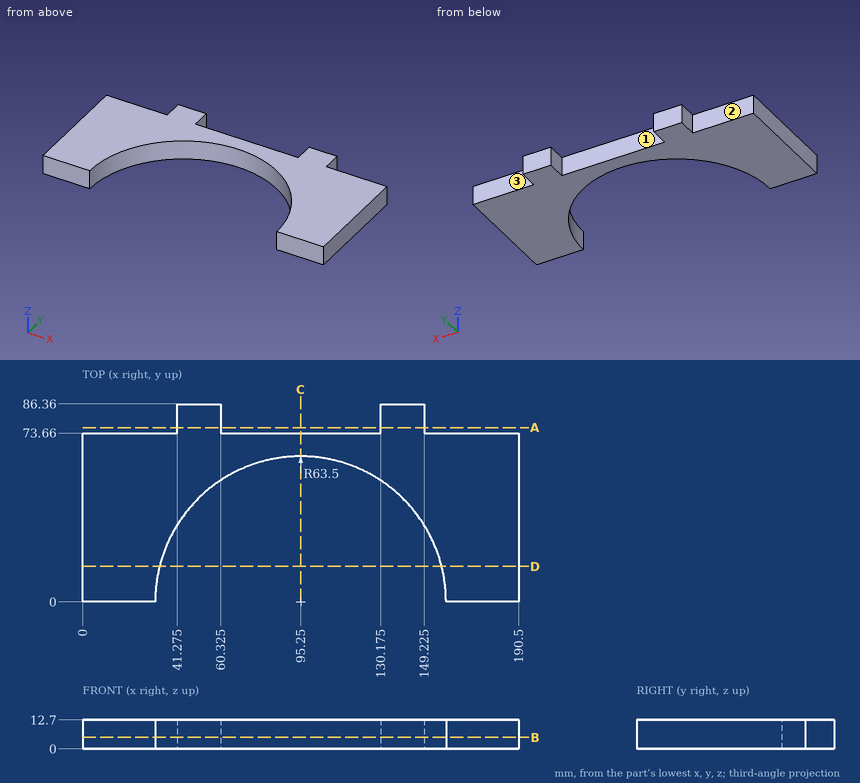
Input: dimensioned drawing with shaded views. Units: mm. Origin: part minimum x, y, z. A direction names the side the tool comes from. Coordinates: 2 decimals unless noted, no trailing zeros. Loops run counter-clockwise (first coordinate to the right, second up) from the corner with the lowest first, then second, coordinate; pieces in that order, holes last. Notation, with made-up numbers: (-24, -15) -> (26, -15) arc R10 cw to (26, 1) -> close; hole circle Ø9 at (55, -21). An arc over 180 degrees is marked (long way). Use a Markdown table: item, result. Add a question column.
(1) Section query C-C, the plane x = 95.25. Return loops of the section in (y, z), plus the area to 3 significant figures.
(2) Section query A-A, the plane y = 76. Return loops of the section in (x, z) (3 decimals).
(3) Section query B-B, the plane z = 5. Return loops of the section in (x, y) (3 decimals).
(4) Line query: line 1 along X through (y, z) = (75, 9.5) (3 decimals); line 2 along X through (y, z) = (15, 10); line 3 along Y through (x, z) = (10.5, 8.5). Output: solid intervals per line, ascending.
(5) Section query D-D, the plane y = 15.5. Return loops of the section in (x, z), plus the area to 3 significant figures.
(6) Access query for the marked faces 1, 2 and 3. Directions: +Z, -Z, +X, -X, +Y, -Y. A direction counts if a zero-diameter tool reaches every point of the face in a straight line with its end or side. Return the directions, or none.
(7) Pin query (flat end, axial travel): pin 1 Ø4 at (x, z) = (14.5, 5) entering from +Y; pin 2 Ø5 at (x, z) = (41.5, 7.5) entering from -Y (3 decimals); pin 3 Ø4 at (y, z) = (77, 7) entering from +X (3 decimals). Return the tip coordinate at first contact, or that it passes through.
Answer:
| question | item | result |
|---|---|---|
| 1 | outline | (63.5, 0) -> (73.66, 0) -> (73.66, 12.7) -> (63.5, 12.7) -> close |
| 1 | area | 129 mm^2 |
| 2 | outline | (41.275, 0) -> (60.325, 0) -> (60.325, 12.7) -> (41.275, 12.7) -> close; (130.175, 0) -> (149.225, 0) -> (149.225, 12.7) -> (130.175, 12.7) -> close |
| 3 | outline | (0, 0) -> (31.75, 0) arc R63.5 cw to (158.75, 0) -> (190.5, 0) -> (190.5, 73.66) -> (149.225, 73.66) -> (149.225, 86.36) -> (130.175, 86.36) -> (130.175, 73.66) -> (60.325, 73.66) -> (60.325, 86.36) -> (41.275, 86.36) -> (41.275, 73.66) -> (0, 73.66) -> close |
| 4 | line 1 | x = 41.275 to 60.325, 130.175 to 149.225 |
| 4 | line 2 | x = 0 to 33.55, 156.95 to 190.5 |
| 4 | line 3 | y = 0 to 73.66 |
| 5 | outline | (0, 0) -> (33.67, 0) -> (33.67, 12.7) -> (0, 12.7) -> close; (156.83, 0) -> (190.5, 0) -> (190.5, 12.7) -> (156.83, 12.7) -> close |
| 5 | area | 855 mm^2 |
| 6 | face 1 | +Z, -Z, +Y |
| 6 | face 2 | +Z, -Z, -X, +Y |
| 6 | face 3 | +Z, -Z, +X, +Y |
| 7 | pin 1 | stops at y = 73.66 |
| 7 | pin 2 | stops at y = 29.465 |
| 7 | pin 3 | stops at x = 149.225 |
